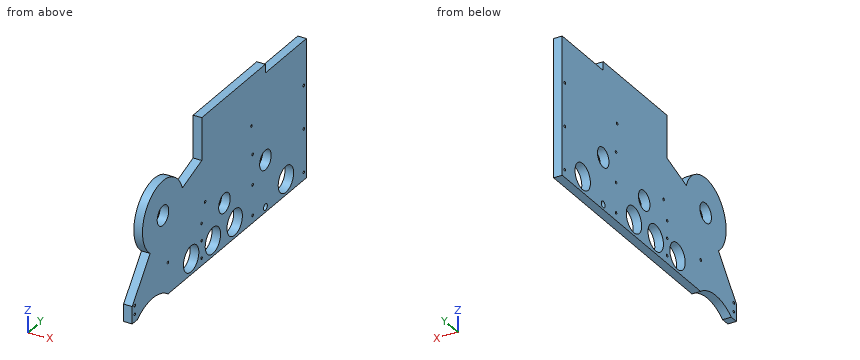
from build123d import *

# Parameters (mm, degrees)
F0_R     = 1.905
F0_R_2   = 14.2875
F0_R_3   = 4.7625
F1_DEPTH = 12.7
F2_R     = 19.05
F3_DEPTH = 12.7
F5_DEPTH = 12.7
F6_R     = 1.905
F7_DEPTH = 12.7


with BuildPart() as f1:
    # F0 (on Right) → F1 (new body)
    with BuildSketch(Plane.YZ):
        with BuildLine():
            Line((0, 355.6), (0, 0))
            Line((0, 0), (12.7, 0))
            ThreePointArc((12.7, 0), (50.8, 12.7), (88.9, 0))
            Line((88.9, 0), (431.8, 0))
            Line((431.8, 0), (431.8, 355.6))
            Line((431.8, 355.6), (0, 355.6))
        make_face()
        with Locations((88.4877131973, 46.0377095938)):
            Circle(F0_R, mode=Mode.SUBTRACT)
        with Locations((180.5685843602, 88.9757249866)):
            Circle(F0_R, mode=Mode.SUBTRACT)
        with Locations((228.6, 63.5)):
            Circle(F0_R_2, mode=Mode.SUBTRACT)
        with Locations((330.2, 7.62)):
            Circle(F0_R_3, mode=Mode.SUBTRACT)
        with Locations((330.2, 76.2)):
            Circle(F0_R_2, mode=Mode.SUBTRACT)
        with Locations((76.2, 120.65)):
            Circle(F0_R_2, mode=Mode.SUBTRACT)
        with Locations((295.6696733139, 142.6482442277)):
            Circle(F0_R, mode=Mode.SUBTRACT)
    extrude(amount=F1_DEPTH)

    # F2 (on face) → F3 (cut, through all)
    with BuildSketch(Plane.YZ.offset(12.7)):
        with Locations((146.05, 23.05)):
            Circle(F2_R)
        with Locations((254, 23.05)):
            Circle(F2_R)
        with Locations((381, 23.0378)):
            Circle(F2_R)
        with Locations((200.025, 23.05)):
            Circle(F2_R)
    extrude(amount=-F3_DEPTH, mode=Mode.SUBTRACT)

    # F4 (on face) → F5 (cut, through all)
    with BuildSketch(Plane.YZ.offset(12.7)):
        Polygon((431.8, 355.6), (0, 355.6), (0, 215.9), (172.3654351189, 215.9), (330.2, 215.9), (355.6, 215.9), (431.8, 215.9), align=None)
        with BuildLine():
            Line((172.3654351189, 215.9), (0, 215.9))
            Line((0, 215.9), (0, 25.4))
            Line((0, 25.4), (44.4654915842, 80.9818644803))
            ThreePointArc((44.4654915842, 80.9818644803), (47.0024645882, 162.2209505049), (124.2827175595, 137.0418355316))
            Line((124.2827175595, 137.0418355316), (172.3654351189, 153.4336710633))
            Line((172.3654351189, 153.4336710633), (172.3654351189, 215.9))
        make_face()
        Polygon((431.8, 203.2), (431.8, 215.9), (355.6, 215.9), (330.2, 207.2409090909), (330.2, 203.2), align=None)
        Polygon((330.2, 207.2409090909), (355.6, 215.9), (330.2, 215.9), align=None)
    extrude(amount=-F5_DEPTH, mode=Mode.SUBTRACT)

    # F6 (on face) → F7 (cut, through all)
    with BuildSketch(Plane.YZ.offset(12.7)):
        with Locations((425.45, 11.1125)):
            Circle(F6_R)
        with Locations((425.45, 74.5109)):
            Circle(F6_R)
        with Locations((425.45, 137.9093)):
            Circle(F6_R)
        with Locations((298.45, 11.1125)):
            Circle(F6_R)
        with Locations((298.45, 100.0125)):
            Circle(F6_R)
        with Locations((298.45, 55.5625)):
            Circle(F6_R)
        with Locations((171.8554794788, 11.1125)):
            Circle(F6_R)
        with Locations((171.8554794788, 36.5125)):
            Circle(F6_R)
        with Locations((171.8554794788, 61.9125)):
            Circle(F6_R)
        with Locations((6.35, 11.1125)):
            Circle(F6_R)
        with Locations((6.35, 23.8125)):
            Circle(F6_R)
    extrude(amount=-F7_DEPTH, mode=Mode.SUBTRACT)


solid = f1.part
Could you check a few things on this model? Use its own coordinates, in mm. Coordinates: 2 decimals unless noted, no trailing zeros. Loops run counter-clockwise (first coordinate to the right, second up) from the corner with the lowest first, then second, coordinate; pieces in that order, holes last. Notation, with made-up numbers: (-25, 68.5) -> (-6, 68.5) arc R18 cw to (-6, 77.5) -> close; hole circle Ø9 at (81, 48). An arc over 180 degrees is marked (long way). Answer in a Markdown table with one row per item.
(1) Imagine slicing it at D-D (z = 183). List the corners of the cut face in (x, y) for me.
Results found:
| item | result |
|---|---|
| outline | (0, 172.37) -> (12.7, 172.37) -> (12.7, 431.8) -> (0, 431.8) -> close |
(2) Imagine slicing it at A-A (y = 381). List the corners of the cut face in (x, z) for me.
Results found:
| item | result |
|---|---|
| outline | (0, 0) -> (12.7, 0) -> (12.7, 3.99) -> (0, 3.99) -> close; (0, 42.09) -> (12.7, 42.09) -> (12.7, 203.2) -> (0, 203.2) -> close |
(3) If I drill on probe 1 along Z at (x, y) = (5.75, 425.45); probe 2 along Z at (x, y) = (10.25, 298.45); probe 3 along Y at (x, z) = (11.25, 35), over which ranges is the centre line in solid material (lowest first)?
Results found:
| item | result |
|---|---|
| probe 1 | z = 0 to 9.21, 13.02 to 72.61, 76.42 to 136, 139.81 to 203.2 |
| probe 2 | z = 0 to 9.21, 13.02 to 53.66, 57.47 to 98.11, 101.92 to 215.9 |
| probe 3 | y = 7.68 to 131.21, 160.89 to 170.7, 173.01 to 185.19, 214.86 to 239.16, 268.84 to 366.17, 395.83 to 431.8 |
(4) Imagine slicing it at C-C (x = 8.25). Give the number of separate pieces and of enclosed holes in the cut face, plus the area to 3 significant figures.
Results found:
| item | result |
|---|---|
| separate pieces | 1 |
| enclosed holes | 22 |
| area | 70,900 mm^2 |
(5) Imagine slicing it at B-B (z = 116). List the corners of the cut face in (x, y) for me, plus the area to 3 significant figures.
Results found:
| item | result |
|---|---|
| outline | (0, 25.61) -> (12.7, 25.61) -> (12.7, 62.69) -> (0, 62.69) -> close; (0, 89.71) -> (12.7, 89.71) -> (12.7, 431.8) -> (0, 431.8) -> close |
| area | 4,820 mm^2 |
